Read the model definition and answer for the solid it produces. Units are mm, in the model's axes. Give positions to 0.01 mm unless a question says otherwise; leave off trailing zeros. Loops run counter-clockwise (first coordinate to the right, second up) from the corner with the lowest first, then second, coordinate; pieces in that order, holes last. Notation, with made-up numbers: (29, -14) - (35, -14) arc R22 ccw to (35, -6) - close; hole circle Ø4 at (64.5, 58). An arc over 180 degrees is marked (long way). Write item = value, one per line.
Autodesk Inventor part; units mm, degrees
ref_plane "YZ Plane" through (0, 0, 0) normal (1, 0, 0) x (0, 1, 0)
ref_plane "XZ Plane" through (0, 0, 0) normal (0, 1, 0) x (-1, 0, 0)
ref_plane "XY Plane" through (0, 0, 0) normal (0, 0, 1) x (1, 0, 0)
sketch "Szkic1" plane through (0, 0, 0) normal (0, 1, 0) x (-1, 0, 0)
  line L0 (0, -1.91) -> (0, -62.23)
  line L1 (0, -62.23) -> (-8.8883, -71.1183)
  line L2 (0, -62.23) -> (12.57, -62.23) construction
  line L3 (-8.8883, -71.1183) -> (-24.1183, -71.1183)
  line L4 (-26.0283, -69.2083) -> (-26.0283, -64.1383)
  line L5 (-24.1183, -62.2283) -> (-12.6883, -62.2283)
  line L6 (-12.6883, -62.2283) -> (-8.877, -58.417)
  line L7 (-12.6883, -62.2283) -> (-7.2983, -62.2283) construction
  line L8 (-8.877, -58.417) -> (-8.877, -1.91)
  line L9 (-6.967, 0) -> (-1.91, 0)
  line L10 (-1.91, 0) -> (0, -1.91)
  line L11 (-8.877, -1.91) -> (-6.967, 0)
  line L12 (-26.0283, -64.1383) -> (-24.1183, -62.2283)
  line L13 (-26.0283, -69.2083) -> (-24.1183, -71.1183)
  line L14 (-26.0283, -66.6733) -> (-15.6934, -66.6733)
  circle A0 centre (-21.5783, -66.6733) radius 0.75
  line L15 (-4.4385, 0) -> (-4.4385, -63.1833)
  circle A1 centre (-4.4385, -6.35) radius 0.75
  circle A2 centre (-4.4385, -21.59) radius 0.75
  circle A3 centre (-4.4385, -36.83) radius 0.75
  circle A4 centre (-4.4385, -52.07) radius 0.75
  line L16 (-1, -61.8158) -> (-1, -2.3242)
  line L17 (-1, -2.3242) -> (-2.3242, -1)
  line L18 (-2.3242, -1) -> (-6.5528, -1)
  line L19 (-6.5528, -1) -> (-7.877, -2.3242)
  line L20 (-7.877, -2.3242) -> (-7.877, -58.8312)
  line L21 (-7.877, -58.8312) -> (-12.2741, -63.2283)
  line L22 (-12.2741, -63.2283) -> (-23.7041, -63.2283)
  line L23 (-23.7041, -63.2283) -> (-25.0283, -64.5525)
  line L24 (-25.0283, -64.5525) -> (-25.0283, -68.7941)
  line L25 (-25.0283, -68.7941) -> (-23.7041, -70.1183)
  line L26 (-23.7041, -70.1183) -> (-9.3025, -70.1183)
  line L27 (-9.3025, -70.1183) -> (-1, -61.8158)
  point P0 (0, 0)
  point P1 (-26.0283, -71.1183)
  point P2 (-26.0283, -62.2283)
  point P3 (-8.877, 0)
  dimension "d0" = 62.23
  dimension "d1" = 135
  dimension "d2" = 12.57
  dimension "d3" = 17.14
  dimension "d4" = 8.89
  dimension "d5" = 13.34
  dimension "d6" = 45
  dimension "d7" = 5.39
  dimension "d8" = 1.91
  dimension "d9" = 1.91
  dimension "d10" = 1.91
  dimension "d11" = 1.91
  dimension "d12" = 1.91
  dimension "d13" = 1.91
  dimension "d14" = 1.91
  dimension "d15" = 1.91
  dimension "d16" = 1.5
  dimension "d17" = 4.45
  dimension "d18" = 1.5
  dimension "d19" = 6.35
  dimension "d22" = 15.24
  dimension "d27" = 19.048
  dimension "d28" = 1
  dimension "d31" = 45.72
extrude "Wyciągnięcie proste1" add sketch "Szkic1" along normal blind 1 contours L18 L17 L16 L27 L26 L25 L24 L23 L22 L21 L20 L19
properties part number "gnd"
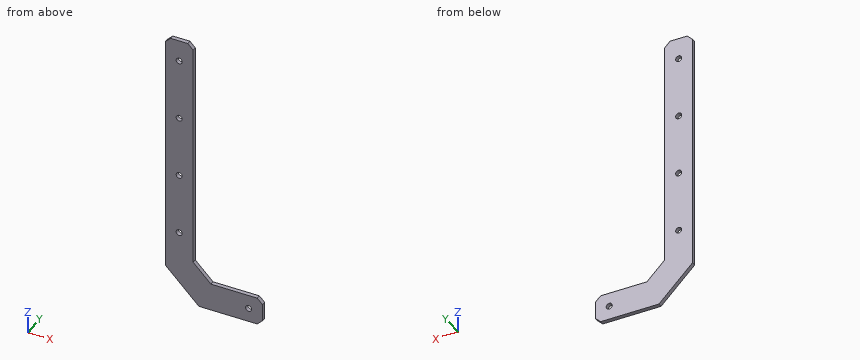
1) A cutting plane is placed at D-D on z = -28.5. Determine the outline of the cut face in (x, y), then the cut area to 3 significant figures.
Output:
outline = (1, 0) - (7.88, 0) - (7.88, 1) - (1, 1) - close
area = 6.88 mm²
2) Each of these flat-tipped pins is pushed along its axis until it touches: P1, Ø8, axis at x = 8, z = -12.5, coming from the -Y side; P2, Ø0.5, axis at x = 18, y = 0.5, coming from the +Z side. Where does it stop, or does it pass through?
Output:
P1 = 0
P2 = -63.23
3) Find the intervals of material crossed by probe 1 along X at (y, z) = (0.6, -36.83); probe 2 along Z at (x, y) = (4.5, 0.05); probe 3 along Z at (x, y) = (4, 0.25), in increasing order.
Output:
probe_1 = 1 to 3.69, 5.19 to 7.88
probe_2 = -65.32 to -52.82, -51.32 to -37.58, -36.08 to -22.34, -20.84 to -7.1, -5.6 to -1
probe_3 = -64.82 to -52.68, -51.46 to -37.44, -36.22 to -22.2, -20.98 to -6.96, -5.74 to -1
4) A cutting plane is placed at B-B on y = 0.5. Determine the outline of the cut face in (x, z).
Output:
outline = (1, -61.82) - (9.3, -70.12) - (23.7, -70.12) - (25.03, -68.79) - (25.03, -64.55) - (23.7, -63.23) - (12.27, -63.23) - (7.88, -58.83) - (7.88, -2.32) - (6.55, -1) - (2.32, -1) - (1, -2.32) - close; hole circle Ø1.5 at (4.44, -52.07); hole circle Ø1.5 at (4.44, -36.83); hole circle Ø1.5 at (4.44, -21.59); hole circle Ø1.5 at (4.44, -6.35); hole circle Ø1.5 at (21.58, -66.67)
5) A cutting plane is placed at A-A on z = -52.07. Determine the outline of the cut face in (x, y).
Output:
outline = (1, 0) - (3.69, 0) - (3.69, 1) - (1, 1) - close; (5.19, 0) - (7.88, 0) - (7.88, 1) - (5.19, 1) - close
6) A cutting plane is placed at C-C on x = 18. Determine the outline of the cut face in (y, z).
Output:
outline = (0, -70.12) - (1, -70.12) - (1, -63.23) - (0, -63.23) - close
